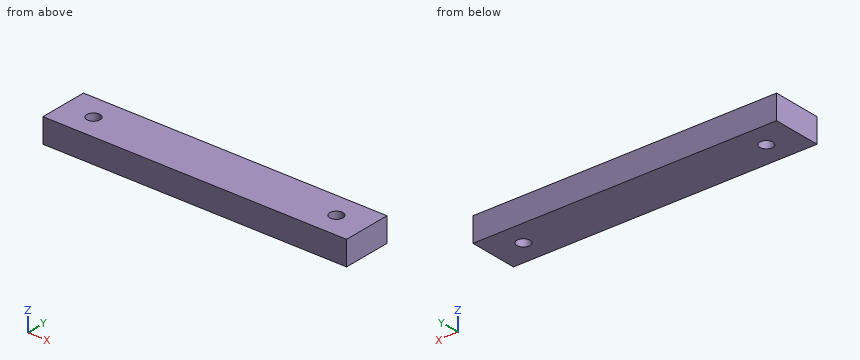
```python
from build123d import *

# Parameters (mm, degrees)
SKETCH2_W               = 150
SKETCH2_H               = 24
BOSS_EXTRUDE1_DEPTH     = 6
CUT_EXTRUDE1_DEPTH      = 77.896033708
CUT_EXTRUDE1_DEPTH_BACK = 77.896033708
SKETCH3_R               = 3.25


with BuildPart() as part:
    # Sketch2 → Boss-Extrude1 (new, symmetric)
    with BuildSketch(Plane.XY):
        Rectangle(SKETCH2_W, SKETCH2_H)
    extrude(amount=BOSS_EXTRUDE1_DEPTH, both=True)

    # Sketch3 → Cut-Extrude1 (cut, two sides: drawn at the far end of the back side and taken through both)
    with BuildSketch(Plane.XY.offset(6).offset(-CUT_EXTRUDE1_DEPTH_BACK)):
        with Locations((-60, 0)):
            Circle(SKETCH3_R)
        with Locations((60, 0)):
            Circle(SKETCH3_R)
    extrude(amount=CUT_EXTRUDE1_DEPTH + CUT_EXTRUDE1_DEPTH_BACK, mode=Mode.SUBTRACT)


solid = part.part
```
Verification items for the finished model (mm, model axes). Coordinates: 2 decimals unless noted, no trailing zeros. Loops run counter-clockwise (first coordinate to the right, second up) from the corner with the lowest first, then second, coordinate; pieces in that order, holes last. Notation, with made-up numbers: (78.25, 6) - (119.25, 6) arc R10 ccw to (119.25, 20) - close; hole circle Ø5 at (88.25, 43.5). An arc over 180 degrees is marked (long way). Return JSON: item names as keys, results as strings.
1. Section check C-C, the plane z = -3.75. Record the boundary of the cut face in (x, y).
Established:
{"outline": "(-75, -12) - (75, -12) - (75, 12) - (-75, 12) - close; hole circle Ø6.5 at (-60, 0); hole circle Ø6.5 at (60, 0)"}
2. Thickness scan on L1, parallel to X at y = 0, z = 2.25; L2, parallel to X at y = 1.5, z = 5.75; L3, parallel to Y at x = -60, z = 2. Record the ranges inside material, lowest first.
Established:
{"L1": "x = -75 to -63.25, -56.75 to 56.75, 63.25 to 75", "L2": "x = -75 to -62.88, -57.12 to 57.12, 62.88 to 75", "L3": "y = -12 to -3.25, 3.25 to 12"}
3. Section check A-A, the plane y = 0. Record the boundary of the cut face in (x, z).
Established:
{"outline": "(-75, -6) - (-63.25, -6) - (-63.25, 6) - (-75, 6) - close; (-56.75, -6) - (56.75, -6) - (56.75, 6) - (-56.75, 6) - close; (63.25, -6) - (75, -6) - (75, 6) - (63.25, 6) - close"}
4. Go/stop test with a flat-tipped pin: pin 1 (7.5 mm diameter, centred on x = -60, y = 0, fed in from -Z). Record where the tip stops, or that it passes through.
Established:
{"pin 1": "stops at z = -6"}
5. Section check B-B, the plane x = -60. Record the boundary of the cut face in (y, z).
Established:
{"outline": "(-12, -6) - (-3.25, -6) - (-3.25, 6) - (-12, 6) - close; (3.25, -6) - (12, -6) - (12, 6) - (3.25, 6) - close"}
